Source: CAD feature listing. Evaluate the final solid. Frame: model axes, mm. Coordinates: 2 decimals unless noted, no trailing zeros. Write each loop counter-clockwise with the first axis right and the second up, starting at its lowest first coordinate (ties: lowest second). Pieces come first, ordered by that corner, then holes. Notation, with made-up numbers: (89, 66.5) -> (148, 66.5) arc R12 ccw to (148, 80.5) -> close; hole circle Ø8 at (-37.75, 20.25). An arc over 180 degrees is marked (long way). Write item = value, one per line.
from build123d import *

# Parameters (mm, degrees)
F0_W      = 450
F0_H      = 200
F1_DEPTH  = 9
F2_W      = 4.5
F2_H      = 200
F3_DEPTH  = 4.5
F4_W      = 4.5
F4_H      = 200
F5_DEPTH  = 4.5
F6_W      = 441
F6_H      = 4.5
F7_DEPTH  = 4.5
F8_W      = 441
F8_H      = 4.5
F9_DEPTH  = 4.5
F10_W     = 395
F10_H     = 121
F11_DEPTH = 9
F12_R     = 2.5
F13_DEPTH = 9


with BuildPart() as f1:
    # F0 (on Right) → F1 (new body)
    with BuildSketch(Plane.YZ):
        Rectangle(F0_W, F0_H)
    extrude(amount=F1_DEPTH)

    # F2 (on face) → F3 (cut)
    with BuildSketch(Plane.XZ.offset(225)):
        with Locations((2.25, 0)):
            Rectangle(F2_W, F2_H)
    extrude(amount=-F3_DEPTH, mode=Mode.SUBTRACT)

    # F4 (on face) → F5 (cut)
    with BuildSketch(Plane(origin=(0, 225, 0), x_dir=(-1, 0, 0), z_dir=(0, 1, 0))):
        with Locations((-2.25, 0)):
            Rectangle(F4_W, F4_H)
    extrude(amount=-F5_DEPTH, mode=Mode.SUBTRACT)

    # F6 (on face) → F7 (cut)
    with BuildSketch(Plane(origin=(0, 0, 0), x_dir=(0, -1, 0), z_dir=(-1, 0, 0))):
        with Locations((0, 52.75)):
            Rectangle(F6_W, F6_H)
    extrude(amount=-F7_DEPTH, mode=Mode.SUBTRACT)

    # F8 (on face) → F9 (cut)
    with BuildSketch(Plane(origin=(0, 0, 0), x_dir=(0, -1, 0), z_dir=(-1, 0, 0))):
        with Locations((0, -52.75)):
            Rectangle(F8_W, F8_H)
    extrude(amount=-F9_DEPTH, mode=Mode.SUBTRACT)

    # F10 (on face) → F11 (cut, through all)
    with BuildSketch(Plane.YZ.offset(9)):
        with Locations((-8, 14.5)):
            Rectangle(F10_W, F10_H)
    extrude(amount=-F11_DEPTH, mode=Mode.SUBTRACT)

    # F12 (on face) → F13 (cut, through all)
    with BuildSketch(Plane.YZ.offset(9)):
        with Locations((-203.5, 84)):
            Circle(F12_R)
        with Locations((171.5, 84)):
            Circle(F12_R)
        with Locations((171.5, -55)):
            Circle(F12_R)
        with Locations((-203.5, -55)):
            Circle(F12_R)
    extrude(amount=-F13_DEPTH, mode=Mode.SUBTRACT)


solid = f1.part
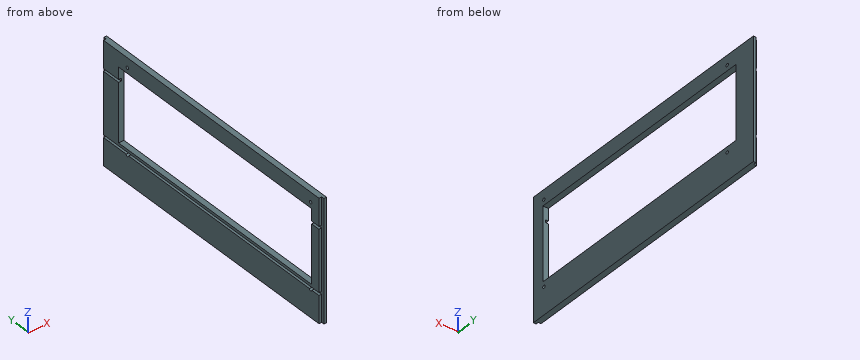
1) Material intervals for probe 1 along Z at (x, y) = (0.75, 82); probe 2 along Z at (x, y) = (3.25, 204); probe 3 along Y at (x, z) = (5.75, -55), sorted ascending. Write a range as [from, to].
Answer block:
probe_1 = [-100, -55], [-50.5, -46], [75, 100]
probe_2 = [-100, -55], [-50.5, 50.5], [55, 100]
probe_3 = [-225, -206], [-201, 169], [174, 225]
2) Cut plane C-C, the plane z = 26.5. Output: boundary loops of the cut face in (x, y), and give its area (4 significant figures).
Answer block:
outline = (0, -220.5) -> (4.5, -220.5) -> (4.5, -225) -> (9, -225) -> (9, -205.5) -> (0, -205.5) -> close; (0, 189.5) -> (9, 189.5) -> (9, 225) -> (4.5, 225) -> (4.5, 220.5) -> (0, 220.5) -> close
area = 454.5 mm2
3) First-contact query: pin 1 Ø3.5 at (x, z) = (1, 75) entering from +Y; pin 2 Ø1.3 at (x, z) = (3.5, -75.5) entering from -Y. Flat tips, straight axial feed; report the tip coordinate or a pass-through.
Answer block:
pin_1 = 220.5
pin_2 = -220.5
4) Cut plane B-B, the plane x = 6.5. Output: boundary loops of the cut face in (y, z), and give its area (3 significant figures).
Answer block:
outline = (-225, -100) -> (225, -100) -> (225, 100) -> (-225, 100) -> close; hole circle Ø5 at (-203.5, -55); hole circle Ø5 at (-203.5, 84); hole (-205.5, -46) -> (189.5, -46) -> (189.5, 75) -> (-205.5, 75) -> close; hole circle Ø5 at (171.5, -55); hole circle Ø5 at (171.5, 84)
area = 42,100 mm2
5) Cut plane A-A, the plane y = -75.5. Output: boundary loops of the cut face in (x, z).
Answer block:
outline = (0, -100) -> (9, -100) -> (9, -46) -> (0, -46) -> (0, -50.5) -> (4.5, -50.5) -> (4.5, -55) -> (0, -55) -> close; (0, 75) -> (9, 75) -> (9, 100) -> (0, 100) -> close
